Source: CAD feature listing. Evaluate the final solid. Frame: model axes, mm. Round coordinates to 2 decimals unless told otherwise and drop trailing zeros. Loops run counter-clockwise (first coordinate to the right, second up) from the corner with the lowest first, then second, coordinate; pieces in that order, holes last. Notation, with made-up numbers: M 56.25,-0.5 L 64.25,-0.5 A5 cw 64.25,7.5 Z; hole C -17.5,68.25 d1. An arc over 180 degrees is marked long. Answer as a JSON object with one key per item and string values.
from build123d import *

# Parameters (mm, degrees)
SKETCH_1_W             = 70
SKETCH_1_H             = 70
SKETCH_1_R             = 8.5
SM_BASE_FLANGE_1_DEPTH = 6


# Sheet-metal steps are written as plain solids
with BuildPart() as part:
    # Sketch 1 → Базовая кромка1 (new body)
    with BuildSketch(Plane(origin=(0, 0, 0), x_dir=(1, 0, 0), z_dir=(0, 1, 0))):
        Rectangle(SKETCH_1_W, SKETCH_1_H)
        with Locations(Location((0, 0, 0), (0, 0, 270))):
            Circle(SKETCH_1_R, mode=Mode.SUBTRACT)
    extrude(amount=-SM_BASE_FLANGE_1_DEPTH)


solid = part.part
Item 1: Section C-C on y = -1.55. Return the cut outline in (x, z).
Answer sheet:
{"outline": "M -35,-35 L 35,-35 L 35,35 L -35,35 Z; hole C 0,0 d17"}
Item 2: Section A-A on z = 0. Return the cut outline in (x, y), then the cut area to 3 significant figures.
Answer sheet:
{"outline": "M -35,-6 L -8.5,-6 L -8.5,0 L -35,0 Z; M 8.5,-6 L 35,-6 L 35,0 L 8.5,0 Z", "area": "318 mm²"}
Item 3: Pull-direction query (Z, two-part tool) for faces 1 (the cylindrical face through (8.428, -2.958, -1.107)), 2 (the flat face through (0, -3, -35)), 3 (the flat face through (7, -6, -8)); classes: pulls with the +Z half, pulls with the -Z half, needs draft (parallel to the pull), parting line crosses it, or undercut.
Answer sheet:
{"face 1": "undercut", "face 2": "pulls with the -Z half", "face 3": "needs draft"}
Item 4: Section B-B on x = 7.5. Return the cut outline in (y, z), then the cut area to 3 significant figures.
Answer sheet:
{"outline": "M -6,-35 L 0,-35 L 0,-4 L -6,-4 Z; M -6,4 L 0,4 L 0,35 L -6,35 Z", "area": "372 mm²"}
Item 5: Line query: probe 1 along X at (y, z) = (-5.1, 0); probe 2 along X at (y, z) = (-2.2, -1.5); probe 3 along Z at (x, y) = (7.5, -3.95). Output: solid intervals per line, ascending. Write a range as from..to.
Answer sheet:
{"probe 1": "x = -35..-8.5, 8.5..35", "probe 2": "x = -35..-8.37, 8.37..35", "probe 3": "z = -35..-4, 4..35"}
